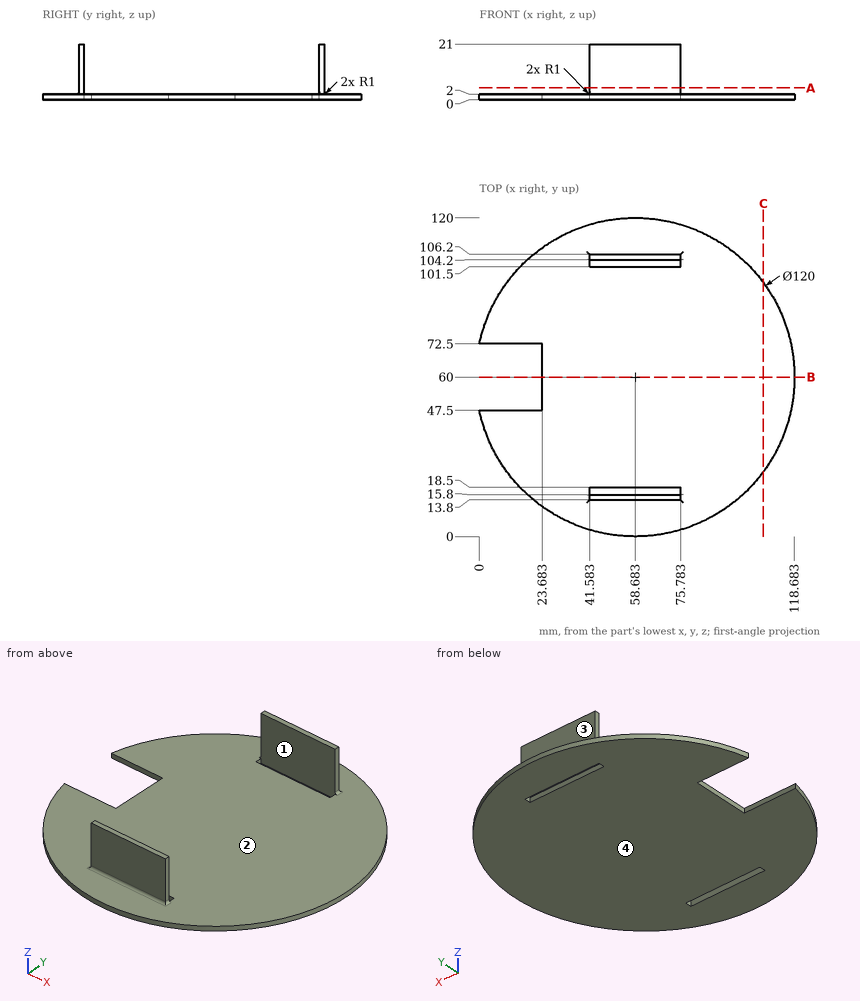
For this review, use the dimensioned drawing (mm, ordinates from the lowest corner) and the shaded views. Coordinates: 2 decimals unless noted, no trailing zeros. Loops run counter-clockwise (first coordinate to the right, second up) from the corner with the lowest first, then second, coordinate; pieces in that order, holes last.
1. Add section C-C, the plane x = 107. Give the boundary of the cut face in (y, z) (1 decimal).
2. Insertion check: P1, Ø0.6, axis at y = 105, z = 8, coming from the +X side; P2, Ø1.6, axis at y = 105, z = 10, coming from the -X side; P3, Ø0.6, axis at y = 102.5, z = 1.5, coming from the +X side (1 decimal); P4, Ø4, axis at x = 101.5, y = 41.5, coming from the -Z side. Each pin has a flat end and moves straight along its axis. Give the tip position at first contact, or say it passes through.
3. Add section B-B, the plane y = 60. Give the boundary of the cut face in (x, z).
4. Mouldability with a two-part tool opening along Y and no side actions: class the marked faces 1, 2, 3 and 4 as +Y half, -Y half, draft (parallel to the pull), parting line (faces both ways), or undercut.
5. Add section A-A, the plane z = 4.5. Give the boundary of the cut face in (x, y).
6. For line 1 (Y direction, x = 56.5, z = 11.5); line 2 (X direction, y = 106, z = 4.5); line 3 (Z direction, x = 49.5, y = 95), list the stretches that pass through material, from the lowest coordinate up.
Result:
1. outline: (24.4, 0) - (95.6, 0) - (95.6, 2) - (24.4, 2) - close
2. P1: stops at x = 75.78
2. P2: stops at x = 41.58
2. P3: stops at x = 101.3
2. P4: stops at z = 0
3. outline: (23.68, 0) - (118.68, 0) - (118.68, 2) - (23.68, 2) - close
4. face 1: undercut
4. face 2: undercut
4. face 3: +Y half
4. face 4: draft
5. outline: (41.58, 13.8) - (75.78, 13.8) - (75.78, 15.8) - (41.58, 15.8) - close; (41.58, 104.2) - (75.78, 104.2) - (75.78, 106.2) - (41.58, 106.2) - close
6. line 1: y = 13.8 to 15.8, 104.2 to 106.2
6. line 2: x = 41.58 to 75.78
6. line 3: z = 0 to 2
